from build123d import *

# Parameters (mm, degrees)
SKETCH_1_R          = 30
SKETCH_1_R_2        = 2.75
EXTRUDE_1_DEPTH     = 5
EXTRUDE_2_DEPTH     = 20
SKETCH_3_R          = 1.5
CUT_EXTRUDE_1_DEPTH = 10


with BuildPart() as part:
    # 草图1 → 凸台-拉伸1 (new body)
    with BuildSketch(Plane.XY):
        Circle(SKETCH_1_R)
        with Locations((0, 22.5)):
            Circle(SKETCH_1_R_2, mode=Mode.SUBTRACT)
        with Locations((19.485571585, 11.25)):
            Circle(SKETCH_1_R_2, mode=Mode.SUBTRACT)
        with Locations((19.485571585, -11.25)):
            Circle(SKETCH_1_R_2, mode=Mode.SUBTRACT)
        with Locations((0, -22.5)):
            Circle(SKETCH_1_R_2, mode=Mode.SUBTRACT)
        with Locations((-19.485571585, -11.25)):
            Circle(SKETCH_1_R_2, mode=Mode.SUBTRACT)
        with Locations((-19.485571585, 11.25)):
            Circle(SKETCH_1_R_2, mode=Mode.SUBTRACT)
    extrude(amount=EXTRUDE_1_DEPTH)

    # 草图2 → 凸台-拉伸2 (add)
    with BuildSketch(Plane.XY.offset(5)):
        with BuildLine():
            Line((-9.367496998, -7.5), (-9.367496998, 7.5))
            ThreePointArc((-9.367496998, 7.5), (12, 0), (-9.367496998, -7.5))
        make_face()
        with BuildLine():
            Line((-3.570714214, 3.5), (-3.570714214, -3.5))
            ThreePointArc((-3.570714214, -3.5), (5, 0), (-3.570714214, 3.5))
        make_face(mode=Mode.SUBTRACT)
    extrude(amount=EXTRUDE_2_DEPTH)

    # 草图3 → 切除-拉伸1 (cut)
    with BuildSketch(Plane.ZY.offset(9.367496998)):
        with Locations((21, 0)):
            Circle(SKETCH_3_R)
        with Locations((15, 0)):
            Circle(SKETCH_3_R)
    extrude(amount=-CUT_EXTRUDE_1_DEPTH, mode=Mode.SUBTRACT)


solid = part.part
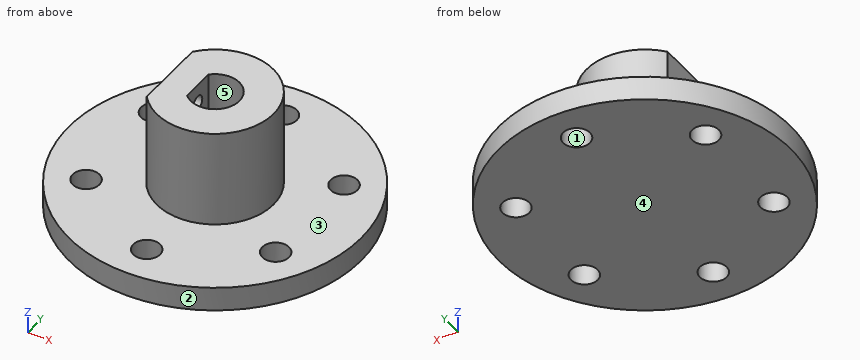
Check sheet for the modelled part. Datum: model origin and axes. Units: mm. Face numbers are marked on the shaded views. A direction names the side the tool comes from. Round coordinates to 2 decimals unless told otherwise and drop trailing zeros. Order: outer loops, then holes, each group sorted by start corner. A loop starts at its lowest first (then second) coordinate and runs counter-clockwise, first axis right, second up.
(1) Access from +Z, -Z, +X, -X, +Y, -Y to the whole of each face (thin tool, end or side, straight path). Record for the marked faces 4 and 5.
(2) Go/stop test with flat-tipped pins: P1, Ø7.5, axis at y = 0, z = 17.5, coming from the -X side; P2, Ø1.8, axis at y = 0, z = 21, coming from the +X side; P3, Ø6.5, axis at x = 19.49, y = 11.25, coming from the +Z side; P4, Ø5, axis at x = 19.49, y = -11.25, coming from the -Z side. Record where each tip stops, or that it passes through.
(3) Cross-section at A-A, the plane y = 0. Enter the section's corners in (x, z).
(4) Cross-section at C-C, the plane x = -1. Enter the section's corners in (y, z).
(5) Draft check along X on the marked faces 1, 2 and 3. Enter one of: pulls with the +X half, pulls with the -X half, needs draft (parallel to the pull), parting line crosses it, or undercut.
(6) Scan lines: probe 1 along Y at (x, z) = (0, 1.7); probe 2 along Z at (x, y) = (-14, 21); probe 3 along X at (y, z) = (21.5, 3). Record each from-to range of solid material in increasing order.
(7) Cross-section at D-D, the plane y = -22.5. Enter the section's corners in (x, z), and give its area (3 significant figures).
(8) Cross-section at B-B, the plane z = 2.75. Enter the section's corners in (x, y).
Check sheet entries:
1. face 4: -Z, +X, -X, +Y, -Y
1. face 5: +Z
2. P1: stops at x = -9.37
2. P2: stops at x = 12
2. P3: stops at z = 5
2. P4: passes through
3. outline: (-30, 0) - (30, 0) - (30, 5) - (12, 5) - (12, 25) - (5, 25) - (5, 5) - (-3.57, 5) - (-3.57, 13.5) - (-9.37, 13.5) - (-9.37, 5) - (-30, 5) - close; (-9.37, 16.5) - (-3.57, 16.5) - (-3.57, 19.5) - (-9.37, 19.5) - close; (-9.37, 22.5) - (-3.57, 22.5) - (-3.57, 25) - (-9.37, 25) - close
4. outline: (-29.98, 0) - (-25.06, 0) - (-25.06, 5) - (-29.98, 5) - close; (-19.94, 0) - (19.94, 0) - (19.94, 5) - (11.96, 5) - (11.96, 25) - (4.9, 25) - (4.9, 5) - (-4.9, 5) - (-4.9, 25) - (-11.96, 25) - (-11.96, 5) - (-19.94, 5) - close; (25.06, 0) - (29.98, 0) - (29.98, 5) - (25.06, 5) - close
5. face 1: undercut
5. face 2: parting line crosses it
5. face 3: needs draft
6. probe 1: y = -30 to -25.25, -19.75 to 19.75, 25.25 to 30
6. probe 2: z = 0 to 5
6. probe 3: x = -20.92 to -2.56, 2.56 to 20.92
7. outline: (-19.84, 0) - (-2.75, 0) - (-2.75, 5) - (-19.84, 5) - close; (2.75, 0) - (19.84, 0) - (19.84, 5) - (2.75, 5) - close
7. area: 171 mm2
8. outline: circle Ø60 at (0, 0); hole circle Ø5.5 at (-19.49, -11.25); hole circle Ø5.5 at (-19.49, 11.25); hole circle Ø5.5 at (0, -22.5); hole circle Ø5.5 at (0, 22.5); hole circle Ø5.5 at (19.49, -11.25); hole circle Ø5.5 at (19.49, 11.25)
